Autodesk Inventor part; units mm, degrees
ref_plane "YZ Plane" through (0, 0, 0) normal (1, 0, 0) x (0, 1, 0)
ref_plane "XZ Plane" through (0, 0, 0) normal (0, 1, 0) x (-1, 0, 0)
ref_plane "XY Plane" through (0, 0, 0) normal (0, 0, 1) x (1, 0, 0)
sketch "Sketch1" plane through (0, 0, 0) normal (1, 0, 0) x (0, 1, 0)
  line L0 (0, 0) -> (-3.175, 0)
  line L1 (-3.175, 0) -> (-3.175, 25.4)
  line L2 (-3.175, 25.4) -> (0, 25.4)
  line L3 (0, 25.4) -> (0, 0)
  line L4 (0, 0) -> (-25.4, 0)
  line L5 (-25.4, 0) -> (-25.4, 3.175)
  line L6 (-25.4, 3.175) -> (0, 3.175)
  line L7 (0, 3.175) -> (0, 0)
  dimension "d0" = 3.175
  dimension "d1" = 25.4
  dimension "d2" = 25.4
  dimension "d3" = 3.175
extrude "Extrusion1" add sketch "Sketch1" along normal blind 660.4
sketch "Sketch2" plane through (0, -25.4, 3.175) normal (0, 0, 1) x (1, 0, 0)
  line L0 (660.4, 22.225) -> (0, 22.225)
  line L1 (0, 22.225) -> (0, 0)
  line L2 (0, 0) -> (660.4, 0)
  line L3 (660.4, 22.225) -> (660.4, 0)
  line L4 (660.4, 0) -> (495.3, 0)
  line L5 (495.3, 0) -> (495.3, 22.225)
  line L6 (495.3, 22.225) -> (660.4, 22.225)
  line L7 (660.4, 22.225) -> (660.4, 0)
  point P0 (0, 25.4)
  dimension "d6" = 165.1
  dimension "d7" = 22.225
extrude "Extrusion2" cut sketch "Sketch2" against normal blind 25.4 contours L3 L2 L5 L0
sketch "Sketch3" plane through (0, 0, 25.4) normal (0, 1, 0) x (1, 0, 0)
  line L0 (0, 25.4) -> (0, 0)
  line L1 (0, 0) -> (660.4, 0)
  line L2 (660.4, 25.4) -> (660.4, 0)
  line L3 (0, 25.4) -> (660.4, 25.4)
  point P0 (647.7, 12.7)
  point P1 (520.7, 12.7)
  point P2 (571.5, 12.7)
  dimension "d10" = 12.7
  dimension "d11" = 12.7
  dimension "d12" = 139.7
  dimension "d13" = 12.7
  dimension "d37" = 88.9
  dimension "d38" = 12.7
sketch "Sketch4" plane through (0, -25.4, 0) normal (0, 0, -1) x (-1, 0, 0)
  line L0 (-660.4, 22.225) -> (-495.3, 22.225)
  line L1 (-495.3, 22.225) -> (-495.3, 0)
  line L2 (0, 0) -> (-495.3, 0)
  line L3 (0, 0) -> (0, 25.4)
  line L4 (0, 25.4) -> (-660.4, 25.4)
  line L5 (-660.4, 22.225) -> (-660.4, 25.4)
  line L6 (0, 0) -> (-495.3, 0)
  line L7 (-495.3, 0) -> (-495.3, 12.7)
  line L8 (-495.3, 12.7) -> (0, 12.7)
  line L9 (0, 12.7) -> (0, 0)
  dimension "d21" = 495.3
  dimension "d22" = 12.7
extrude "Extrusion3" cut sketch "Sketch4" against normal blind 25.4 contours L8 L3 L2 L1
sketch "Sketch5" plane through (0, 0, 25.4) normal (0, 1, 0) x (1, 0, 0)
  line L0 (0, 25.4) -> (0, 0)
  line L1 (0, 0) -> (660.4, 0)
  line L2 (660.4, 25.4) -> (660.4, 0)
  line L3 (0, 25.4) -> (660.4, 25.4)
  point P0 (12.7, 12.7)
  dimension "d25" = 12.7
  dimension "d26" = 12.7
hole "Hole2" at (12.7, 0, 12.7) direction (0, -1, 0) diameter 12.7 end through all
pattern_linear "Rectangular Pattern1" count 19 spacing 25.4 along (1, 0, 0) of "Hole2"
hole "Hole3" at (647.7, 0, 12.7) at (520.7, 0, 12.7) at (571.5, 0, 12.7) direction (0, -1, 0) diameter 6.7469 end through all
properties part number "bottom clamper arm" material "Aluminum 6061"
The listing builds one solid part. Answer for the finished solid, in the listing's coordinates (mm). Coordinates: 2 decimals unless noted, no trailing zeros. Write each loop counter-clockwise with the first axis right and the second up, starting at its lowest first coordinate (ties: lowest second). Pieces come first, ordered by that corner, then holes. Notation, with made-up numbers: (12.25, -8.5) -> (38.25, -8.5) arc R5 cw to (38.25, 0.5) -> close; hole circle Ø9 at (41, 52). An arc over 180 degrees is marked (long way). Write each question's results on one line, items separated by ' | '. Start each with the question number.
1) A cutting plane is placed at A-A (x = 215.9). Determine the outline of the cut face in (y, z) (3 decimals).
2) A cutting plane is placed at B-B (y = -9). Determine the outline of the cut face in (x, z) (3 decimals).
3) A cutting plane is placed at C-C (x = 549). Determine the outline of the cut face in (y, z) (3 decimals).
4) Flat-ended cylindrical pins translate along their axes: pin 1 Ø2 at (x, z) = (170, 4.5) entering from -Y (3 decimals); pin 2 Ø2.5 at (y, z) = (-10, 1.5) entering from +X. Find the tip coordinate at first contact, or state that the pin passes through.
5) Straight lines are drawn through the part: probe 1 along Z at (x, y) = (190.5, -0.65); probe 2 along Y at (x, z) = (617, 16) (3 decimals); probe 3 along Z at (x, y) = (303.5, -4.5) (3 decimals). For each, find the intervals that lie inside material, in ascending order.
6) For a pull along Z with two mould halves and no side action, classify faces 1 (the flat face through (252, -6, 0)), 2 (the flat face through (326, 0, 13)), 3 (the cylindrical face through (450.7, -1.61, 11.32)) as +Z half, -Z half, draft (parallel to the pull), parting line (faces both ways), or undercut.
Values follow:
1) outline: (-12.7, 0) -> (0, 0) -> (0, 6.35) -> (-3.175, 6.35) -> (-3.175, 3.175) -> (-12.7, 3.175) -> close; (-3.175, 19.05) -> (0, 19.05) -> (0, 25.4) -> (-3.175, 25.4) -> close
2) outline: (0, 0) -> (495.3, 0) -> (495.3, 3.175) -> (0, 3.175) -> close
3) outline: (-3.175, 0) -> (0, 0) -> (0, 25.4) -> (-3.175, 25.4) -> close
4) pin 1: y = -3.175 | pin 2: x = 495.3
5) probe 1: 0 to 6.35, 19.05 to 25.4 | probe 2: -3.175 to 0 | probe 3: 0 to 3.175
6) face 1: -Z half | face 2: draft | face 3: undercut
